Can you work these out from the model? Positions are in its coordinate system, mm. A direction names the side the tool comes from. Give positions to 0.01 mm unless a question says otherwise; leave off trailing zeros. Loops run counter-clockwise (first coordinate to the right, second up) from the corner with the lowest first, then second, coordinate; pieces in that order, holes last. Notation, with made-up numbers: (-32.75, 13.5) -> (-25.75, 13.5) arc R9 cw to (-25.75, 19.5) -> close; hole circle Ø1 at (20.25, 86). An arc over 180 degrees is marked (long way). One line per question, with ' | ' between items.
from build123d import *

# Parameters (mm, degrees)
F1_DEPTH  = 2
F2_DEPTH  = 9
F3_W      = 2
F3_H      = 5
F3_H_2    = 4
F4_DEPTH  = 5
F5_W      = 2
F5_H      = 5
F6_DEPTH  = 5
F7_R      = 1.2
F8_DEPTH  = 40
F11_DEPTH = 1
F12_W     = 5
F12_H     = 2
F12_H_2   = 0.5
F13_DEPTH = 2
F14_SIZE  = 1.99999
F12_W_2   = 0.5
F15_DEPTH = 3


# Not quite as in the source:
# - a fillet or chamfer is up to 0.001 mm smaller than in the source, because OpenCascade refuses the exact size


with BuildPart() as f1:
    # F0 (on Top) → F1 (new body)
    with BuildSketch(Plane.XY):
        Polygon((-5.1606558692, 9.7513413054), (-11.6606558692, 9.7513413054), (-11.6606558692, -27.7486586946), (-5.1606558692, -27.7486586946), (2.8393441308, -27.7486586946), (9.3393441308, -27.7486586946), (9.3393441308, 9.7513413054), (2.8393441308, 9.7513413054), align=None)
        Polygon((-9.6606558692, -1.2486586946), (-9.6606558692, 7.7513413054), (7.3393441308, 7.7513413054), (7.3393441308, -1.2486586946), (7.3393441308, -16.7486586946), (7.3393441308, -25.7486586946), (-9.6606558692, -25.7486586946), (-9.6606558692, -16.7486586946), align=None, mode=Mode.SUBTRACT)
        with BuildLine():
            Line((7.3393441308, 7.7513413054), (-9.6606558692, 7.7513413054))
            Line((-9.6606558692, 7.7513413054), (-9.6606558692, -1.2486586946))
            Line((-9.6606558692, -1.2486586946), (-5.6339097184, -1.2486586946))
            ThreePointArc((-5.6339097184, -1.2486586946), (-2.8409986659, 7.1883679509), (4.3393441308, 1.9513413054))
            ThreePointArc((4.3393441308, 1.9513413054), (4.0763707763, 0.2709985087), (3.3125979801, -1.2486586946))
            Line((3.3125979801, -1.2486586946), (7.3393441308, -1.2486586946))
            Line((7.3393441308, -1.2486586946), (7.3393441308, 7.7513413054))
        make_face()
        with BuildLine():
            Line((-5.6339097184, -16.7486586946), (-9.6606558692, -16.7486586946))
            Line((-9.6606558692, -16.7486586946), (-9.6606558692, -25.7486586946))
            Line((-9.6606558692, -25.7486586946), (7.3393441308, -25.7486586946))
            Line((7.3393441308, -25.7486586946), (7.3393441308, -16.7486586946))
            Line((7.3393441308, -16.7486586946), (3.3125979801, -16.7486586946))
            ThreePointArc((3.3125979801, -16.7486586946), (4.0763707763, -18.2683158979), (4.3393441308, -19.9486586946))
            ThreePointArc((4.3393441308, -19.9486586946), (-2.8409986659, -25.1856853401), (-5.6339097184, -16.7486586946))
        make_face()
    extrude(amount=F1_DEPTH)

    # F0 (on Top) → F2 (join)
    with BuildSketch(Plane.XY):
        Polygon((-5.1606558692, 9.7513413054), (-11.6606558692, 9.7513413054), (-11.6606558692, -27.7486586946), (-5.1606558692, -27.7486586946), (2.8393441308, -27.7486586946), (9.3393441308, -27.7486586946), (9.3393441308, 9.7513413054), (2.8393441308, 9.7513413054), align=None)
        Polygon((-9.6606558692, -1.2486586946), (-9.6606558692, 7.7513413054), (7.3393441308, 7.7513413054), (7.3393441308, -1.2486586946), (7.3393441308, -16.7486586946), (7.3393441308, -25.7486586946), (-9.6606558692, -25.7486586946), (-9.6606558692, -16.7486586946), align=None, mode=Mode.SUBTRACT)
    extrude(amount=F2_DEPTH)

    # F3 (on face) → F4 (join)
    with BuildSketch(Plane(origin=(-11.6606558692, 0, 0), x_dir=(0, -1, 0), z_dir=(-1, 0, 0))):
        with Locations((-8.7513413054, 2.5)):
            Rectangle(F3_W, F3_H)
        with Locations((-8.7513413054, 7)):
            Rectangle(F3_W, F3_H_2)
        with Locations((26.7486586946, 2.5)):
            Rectangle(F3_W, F3_H)
        with Locations((26.7486586946, 7)):
            Rectangle(F3_W, F3_H_2)
    extrude(amount=F4_DEPTH)

    # F5 (on face) → F6 (join)
    with BuildSketch(Plane.YZ.offset(9.3393441308)):
        with Locations((-26.7486586946, 2.5)):
            Rectangle(F5_W, F5_H)
        with Locations((8.7513413054, 2.5)):
            Rectangle(F5_W, F5_H)
    extrude(amount=F6_DEPTH)

    # F7 (on face) → F8 (cut)
    with BuildSketch(Plane.XZ.offset(27.7486586946)):
        with Locations((-13.6606558692, 2.6015837211)):
            Circle(F7_R)
        with Locations((11.3393441308, 2.6015837211)):
            Circle(F7_R)
        with Locations((-13.6606558692, 6.9661107846)):
            Circle(F7_R)
    extrude(amount=-F8_DEPTH, mode=Mode.SUBTRACT)

    # F10 (on offset) → F11 (join, symmetric)
    with BuildSketch(Plane(origin=(0, -10.2486586946, 0), x_dir=(-1, 0, 0), z_dir=(0, 1, 0))):
        Polygon((-13.3393441308, 4), (-13.3393441308, 0), (-9.3393441308, 0), (-9.3393441308, 2), (-11.3393441308, 2), (-11.3393441308, 4), align=None)
    extrude(amount=F11_DEPTH, both=True)

    # F12 (on face) → F13 (join)
    with BuildSketch(Plane.XY.offset(9)):
        with Locations((-1.1606558692, -26.7486586946)):
            Rectangle(F12_W, F12_H)
        with Locations((-1.1606558692, -25.4986586946)):
            Rectangle(F12_W, F12_H_2)
        with Locations((-1.1606558692, 8.7513413054)):
            Rectangle(F12_W, F12_H)
        with Locations((-1.1606558692, 7.5013413054)):
            Rectangle(F12_W, F12_H_2)
    extrude(amount=F13_DEPTH)

    # F14 (size 2 in the source; OpenCascade refuses exactly that, so slightly less here)
    f14_edges = [f1.edges().sort_by_distance(p)[0] for p in [
        (-1.160656, -25.248659, 11),
        (-1.160656, 7.251341, 11),
    ]]
    chamfer(f14_edges, length=F14_SIZE)

    # F12 (on face) → F15 (cut)
    with BuildSketch(Plane.XY.offset(9)):
        with Locations((-3.9106558692, -26.7486586946)):
            Rectangle(F12_W_2, F12_H)
        with Locations((1.5893441308, -26.7486586946)):
            Rectangle(F12_W_2, F12_H)
        with Locations((1.5893441308, 8.7513413054)):
            Rectangle(F12_W_2, F12_H)
        with Locations((-3.9106558692, 8.7513413054)):
            Rectangle(F12_W_2, F12_H)
    extrude(amount=-F15_DEPTH, mode=Mode.SUBTRACT)


solid = f1.part
Q1. If we section it at D-D (x = 12): Write out the boundary of the cut face in (y, z), plus the area to 3 significant figures.
Entries:
outline: (-27.75, 0) -> (-25.75, 0) -> (-25.75, 1.6) -> (-27.75, 1.6) -> close; (-27.75, 3.6) -> (-25.75, 3.6) -> (-25.75, 5) -> (-27.75, 5) -> close; (-11.25, 0) -> (-9.25, 0) -> (-9.25, 4) -> (-11.25, 4) -> close; (7.75, 0) -> (9.75, 0) -> (9.75, 1.6) -> (7.75, 1.6) -> close; (7.75, 3.6) -> (9.75, 3.6) -> (9.75, 5) -> (7.75, 5) -> close | area: 20.0 mm²
Q2. If we section it at A-A (y = -16): Write out the boundary of the cut face in (x, z), plus the area to 3 significant figures.
Entries:
outline: (-11.66, 0) -> (-9.66, 0) -> (-9.66, 9) -> (-11.66, 9) -> close; (7.34, 0) -> (9.34, 0) -> (9.34, 9) -> (7.34, 9) -> close | area: 36.0 mm²
Q3. If I drill on probe 1 along Y at (x, z) = (3, 5.5); probe 2 along X at (y, z) = (6, 8.75); probe 3 along Y at (x, z) = (-6, 0.75), over which ranges is the centre line in solid material (lowest first)? Write a range as from..to.
Entries:
probe 1: -27.75..-25.75, 7.75..9.75 | probe 2: -11.66..-9.66, 7.34..9.34 | probe 3: -27.75..-22.56, -17.34..-16.75, -1.25..-0.66, 4.56..9.75
Q4. For pin 1 Ø12.5 at (x, y) = (-1.16, 1.95) entering from +Z; pin 2 Ø1.2 at (y, z) = (9, 8.5) entering from +X; pin 3 Ø4.5 at (y, z) = (-9.5, 2.5) entering from +X; pin 4 Ø2 at (x, z) = (-13.66, 2.6) entering from -Y, each with a flat end and sliding along its axis, tell me the tip position at first contact or that it passes through.
Entries:
pin 1: z = 9.95 | pin 2: x = 9.34 | pin 3: x = 13.34 | pin 4: through
Q5. If we mould it in two halves opening along Z, with no side actions, what happens to faces 5 (the face through (6, -18, 0)), 6 (the face through (-4.161, -27, 8)), 7 (the face through (-1, -25.749, 5))? For each: pulls with the +Z half, pulls with the -Z half, needs draft (parallel to the pull), parting line crosses it, or undercut.
Entries:
face 5: pulls with the -Z half | face 6: needs draft | face 7: undercut
Q6. If we section it at B-B (z = 1): Write out the boundary of the cut face in (x, y).
Entries:
outline: (-16.66, -27.75) -> (14.34, -27.75) -> (14.34, -25.75) -> (9.34, -25.75) -> (9.34, -11.25) -> (13.34, -11.25) -> (13.34, -9.25) -> (9.34, -9.25) -> (9.34, 7.75) -> (14.34, 7.75) -> (14.34, 9.75) -> (-16.66, 9.75) -> (-16.66, 7.75) -> (-11.66, 7.75) -> (-11.66, -25.75) -> (-16.66, -25.75) -> close; hole (-9.66, -16.75) -> (-5.63, -16.75) arc R5.5 ccw (long way) to (3.31, -16.75) -> (7.34, -16.75) -> (7.34, -1.25) -> (3.31, -1.25) arc R5.5 ccw (long way) to (-5.63, -1.25) -> (-9.66, -1.25) -> close
Q7. On a 3-axis mill with a long thin cutter (end or side, diameter ignored), from which of +Z, -Z, +X, -X, +Y, -Y can I reach the whole of each face in a straight line? I mean faces 1 (the face through (-4.161, 9, 8)), 2 (the face through (8, -8, 9)), 3 (the face through (-13.02, 8.74, 7.98)), 4 (the face through (-14, -25.749, 5)). Say none if no direction works.
Entries:
face 1: +Z, +Y, -Y | face 2: +Z, +X, +Y, -Y | face 3: +Y, -Y | face 4: +Z, -Z, -X
